Design review of the part built by this model. Coordinates are the model's own, in mm. A direction names the side the tool comes from. Coordinates: 2 decimals unless noted, no trailing zeros. Loops run counter-clockwise (first coordinate to the right, second up) from the corner with the lowest first, then second, coordinate; pieces in that order, holes last. Notation, with made-up numbers: (-10.5, 43.5) -> (24.5, 43.5) arc R24 ccw to (24.5, 60.5) -> close; hole circle Ø7 at (71.25, 7). An arc over 180 degrees is marked (long way). Use CSV: the item, a comma, the result in double quotes.
```python
from build123d import *

# Parameters (mm, degrees)
SKETCH1_W           = 66.04
SKETCH1_H           = 60.96
SKETCH1_R           = 3.949643495
SKETCH1_R_2         = 4.169884911
SKETCH1_R_3         = 4.009399438
BOSS_EXTRUDE1_DEPTH = 7.62
SKETCH3_W           = 66.04
SKETCH3_H           = 19.05
BOSS_EXTRUDE2_DEPTH = 92.71
SKETCH4_W           = 66.04
SKETCH4_H           = 15.875
BOSS_EXTRUDE3_DEPTH = 50.8
SKETCH5_R           = 15.875
CUT_EXTRUDE2_DEPTH  = 15.875
FILLET1_R           = 12.7
CHAMFER2_SIZE       = 2.54
CHAMFER3_SIZE       = 13.97


with BuildPart() as part:
    # Sketch1 → Boss-Extrude1 (new body)
    with BuildSketch(Plane(origin=(0, 0, 0), x_dir=(1, 0, 0), z_dir=(0, 1, 0))):
        with Locations((-10.475534623, -61.030768925)):
            Rectangle(SKETCH1_W, SKETCH1_H)
        with Locations((-32.891034623, -79.700340115)):
            Circle(SKETCH1_R, mode=Mode.SUBTRACT)
        with Locations((11.939965377, -79.700340115)):
            Circle(SKETCH1_R_2, mode=Mode.SUBTRACT)
        with Locations((-10.475534623, -55.697340115)):
            Circle(SKETCH1_R_3, mode=Mode.SUBTRACT)
    extrude(amount=BOSS_EXTRUDE1_DEPTH)

    # Sketch3 → Boss-Extrude2 (add)
    with BuildSketch(Plane(origin=(0, 7.62, 0), x_dir=(1, 0, 0), z_dir=(0, 1, 0))):
        with Locations((-10.475534623, -40.075768925)):
            Rectangle(SKETCH3_W, SKETCH3_H)
    extrude(amount=BOSS_EXTRUDE2_DEPTH)

    # Sketch4 → Boss-Extrude3 (add)
    with BuildSketch(Plane.XY.offset(49.600768925)):
        with Locations((-10.475534623, 92.3925)):
            Rectangle(SKETCH4_W, SKETCH4_H)
    extrude(amount=BOSS_EXTRUDE3_DEPTH)

    # Sketch5 → Cut-Extrude2 (cut)
    with BuildSketch(Plane(origin=(0, 100.33, 0), x_dir=(1, 0, 0), z_dir=(0, 1, 0))):
        with Locations((-10.475534623, -75.000768925)):
            Circle(SKETCH5_R)
    extrude(amount=-CUT_EXTRUDE2_DEPTH, mode=Mode.SUBTRACT)

    # Fillet1
    fillet1_edges = [part.edges().sort_by_distance(p)[0] for p in [
        (-10.475534623, 100.33, 30.550768925),
    ]]
    fillet(fillet1_edges, radius=FILLET1_R)

    # Chamfer2
    chamfer2_edges = [part.edges().sort_by_distance(p)[0] for p in [
        (-43.495534623, 7.62, 70.555768925),
        (22.544465377, 100.33, 71.825768925),
        (22.544465377, 46.0375, 49.600768925),
        (-43.495534623, 46.0375, 49.600768925),
        (-10.475534623, 7.62, 91.510768925),
        (-43.495534623, 84.455, 75.000768925),
        (22.544465377, 84.455, 75.000768925),
        (-43.495534623, 100.33, 71.825768925),
        (-43.495534623, 43.815, 30.550768925),
        (-43.495534623, 96.610256121, 34.270512804),
        (22.544465377, 43.815, 30.550768925),
        (22.544465377, 96.610256121, 34.270512804),
        (22.544465377, 7.62, 70.555768925),
    ]]
    chamfer(chamfer2_edges, length=CHAMFER2_SIZE)

    # Chamfer3
    chamfer3_edges = [part.edges().sort_by_distance(p)[0] for p in [
        (-43.495534623, 92.3925, 100.400768925),
        (22.544465377, 92.3925, 100.400768925),
    ]]
    chamfer(chamfer3_edges, length=CHAMFER3_SIZE)


solid = part.part
```
Item 1: Clearance check with flat-ended pins moving along their axes: pin 1 (4 mm diameter, centred on x = -22.5, y = 3.5, fed in from +Z); pin 2 (7.5 mm diameter, centred on x = 11.94, z = 79.7, fed in from -Y) (3 decimals). State where each tip first meets the part, or that it passes through.
Checked values:
pin 1,"z = 91.51"
pin 2,"y = 84.455"
Item 2: Add section B-B (y = 11). Give the boundary of the cut face in (x, z).
Checked values:
outline,"(-43.5, 33.09) -> (-40.96, 30.55) -> (20, 30.55) -> (22.54, 33.09) -> (22.54, 47.06) -> (20, 49.6) -> (-40.96, 49.6) -> (-43.5, 47.06) -> close"
Item 3: To check wall thickness, follow line 1 along Y through (x, z) = (-31, 72) (3 decimals); line 2 along Z through (x, y) = (-6, 43.5); line 3 along X through (y, z) = (84.5, 67). State the ranges of each line that lie inside material, in increasing order.
Checked values:
line 1,"0 to 7.62, 84.455 to 100.33"
line 2,"30.55 to 49.6"
line 3,"-41 to -24.19, 3.24 to 20.05"
Item 4: Add section D-D (x = -12). Give the boundary of the cut face in (y, z) (3 decimals).
Checked values:
outline,"(0, 30.551) -> (87.63, 30.551) arc R12.7 ccw to (100.33, 43.251) -> (100.33, 59.199) -> (84.455, 59.199) -> (84.455, 49.601) -> (7.62, 49.601) -> (7.62, 51.989) -> (0, 51.989) -> close; (0, 59.406) -> (7.62, 59.406) -> (7.62, 88.971) -> (5.08, 91.511) -> (0, 91.511) -> close; (84.455, 90.802) -> (100.33, 90.802) -> (100.33, 100.401) -> (84.455, 100.401) -> close"
Item 5: Add section C-C (z = 65). Give the boundary of the cut face in (x, y) (3 decimals).
Checked values:
outline,"(-43.496, 0) -> (22.544, 0) -> (22.544, 5.08) -> (20.004, 7.62) -> (-40.956, 7.62) -> (-43.496, 5.08) -> close; (-43.496, 86.995) -> (-40.956, 84.455) -> (-22.804, 84.455) -> (-22.804, 100.33) -> (-40.956, 100.33) -> (-43.496, 97.79) -> close; (1.853, 84.455) -> (20.004, 84.455) -> (22.544, 86.995) -> (22.544, 97.79) -> (20.004, 100.33) -> (1.853, 100.33) -> close"
Item 6: Draft analysis for pull direction X (two halves, no side actions). For faces 1 (the face through (21.29, 85.74, 67.72)), 2 (the face through (-33.405, 3.757, 75.784)), 3 (the face through (-11, 7.62, 69)), 4 (the face through (11.397, 3.757, 75.566)), state which applies: pulls with the +X half, pulls with the -X half, needs draft (parallel to the pull), parting line crosses it, or undercut.
Checked values:
face 1,"pulls with the +X half"
face 2,"undercut"
face 3,"needs draft"
face 4,"undercut"
Item 7: Add section A-A (x = 11). Give the boundary of the cut face in (y, z) (3 decimals).
Checked values:
outline,"(0, 30.551) -> (87.63, 30.551) arc R12.7 ccw to (100.33, 43.251) -> (100.33, 97.975) -> (84.455, 97.975) -> (84.455, 49.601) -> (7.62, 49.601) -> (7.62, 75.638) -> (0, 75.638) -> close; (0, 83.763) -> (7.62, 83.763) -> (7.62, 88.971) -> (5.08, 91.511) -> (0, 91.511) -> close"
Item 8: Machinability: for faces 5 (the face through (-42.208, 6.368, 69.597)), 6 (the face through (21.292, 45.464, 48.313)), 7 (the face through (-36.413, 92.281, 93.514)), 8 (the face through (-11, 3, 91.511)), 9 (the face through (15.657, 92.281, 93.318)), which of the approach directions +Z, -Z, +X, -X, +Y, -Y give a long, thin tool a straight path to every point of the face, cutting with its end or side? Answer none if there is none.
Checked values:
face 5,"+Z, -X"
face 6,"+Z, +X"
face 7,"+Z, -X, +Y"
face 8,"+Z, +X, -X, -Y"
face 9,"+Z, +X, +Y"
